from build123d import *

# Parameters (mm, degrees)
F1_R     = 16.141204
F2_DEPTH = 3
F3_DEPTH = 25


with BuildPart() as f2:
    # F1 (on Front) → F2 (new body)
    with BuildSketch(Plane.XZ):
        Circle(F1_R)
    extrude(amount=F2_DEPTH)

    # F0 (on Front) → F3 (cut)
    with BuildSketch(Plane.XZ):
        Polygon((3.743937, -6.438396), (7.447783, 0.023146), (3.703846, 6.461542), (-3.743937, 6.438396), (-7.447783, -0.023146), (-3.703846, -6.461542), align=None)
    extrude(amount=F3_DEPTH, mode=Mode.SUBTRACT)


solid = f2.part
The model under review builds one solid part; all positions refer to its coordinate system, in mm. A direction names the side the tool comes from. Give positions to 0.01 mm unless a question says otherwise; leave off trailing zeros. Loops run counter-clockwise (first coordinate to the right, second up) from the corner with the lowest first, then second, coordinate; pieces in that order, holes last. Notation, with made-up numbers: (-28, 57) -> (28, 57) arc R18 cw to (28, 76) -> close; hole circle Ø4 at (-29.75, 38). An arc over 180 degrees is marked (long way). Write each question's results on one line, items separated by ' | '.
1) Take a section at D-D, the plane z = -7.5. Give the boundary of the cut face in (x, y).
Conclusion:
outline: (-14.29, -3) -> (14.29, -3) -> (14.29, 0) -> (-14.29, 0) -> close
2) Draft analysis for pull direction Z (two halves, no side actions). For faces 1 (the face through (-5.57, -1.48, 3.25)), 2 (the face through (-3.499, -1.479, -15.757)), 3 (the face through (0, -3, -7)), state which applies: pulls with the +Z half, pulls with the -Z half, needs draft (parallel to the pull), parting line crosses it, or undercut.
Conclusion:
face 1: undercut | face 2: parting line crosses it | face 3: needs draft
3) For line 1 along Z through (x, y) = (-3, -2.05); line 2 along X through (y, z) = (-1.1, -4.5); line 3 along X through (y, z) = (-0.5, 1.5), list the stretches that pass through material, from the lowest coordinate up. Write a range as from..to.
Conclusion:
line 1: z = -15.86..-6.46, 6.44..15.86 | line 2: x = -15.5..-4.84, 4.86..15.5 | line 3: x = -16.07..-6.57, 6.59..16.07
4) Tool access review of faces 4 (the face through (5.57, -1.48, -3.25)), 5 (the face through (0, 0, -7)): name each direction out of +Z, -Z, +X, -X, +Y, -Y from which nothing blocks a thin tool from reaching the whole face with its end or side.
Conclusion:
face 4: +Y, -Y | face 5: +Z, -Z, +X, -X, +Y
5) Take a section at B-B, the plane x = 0. Give the boundary of the cut face in (y, z).
Conclusion:
outline: (-3, -16.14) -> (0, -16.14) -> (0, -6.45) -> (-3, -6.45) -> close; (-3, 6.45) -> (0, 6.45) -> (0, 16.14) -> (-3, 16.14) -> close
6) Insertion check: pin 1 Ø1 at (x, y) = (2.5, -2) entering from +Z; pin 2 Ø1.5 at (y, z) = (-1, 2) entering from -X; pin 3 Ø1 at (x, y) = (-12.5, -1) entering from +Z; pin 4 Ø2 at (x, z) = (6, 3.5) entering from +Y. Each pin has a flat end and moves straight along its axis. Give the tip position at first contact, or say it passes through.
Conclusion:
pin 1: stops at z = 16.02 | pin 2: stops at x = -16.09 | pin 3: stops at z = 10.8 | pin 4: stops at y = 0
7) Take a section at A-A, the plane y = -2.15. Give the boundary of the cut face in (x, z), plus the area to 3 significant figures.
Conclusion:
outline: circle Ø32.28 at (0, 0); hole (-7.45, -0.02) -> (-3.7, -6.46) -> (3.74, -6.44) -> (7.45, 0.02) -> (3.7, 6.46) -> (-3.74, 6.44) -> close | area: 674 mm^2
8) Take a section at C-C, the plane x = -7. Give the boundary of the cut face in (y, z).
Conclusion:
outline: (-3, -14.54) -> (0, -14.54) -> (0, -0.79) -> (-3, -0.79) -> close; (-3, 0.76) -> (0, 0.76) -> (0, 14.54) -> (-3, 14.54) -> close
